from build123d import *

# Parameters (mm, degrees)
F0_R     = 2.5
F0_W     = 45
F0_H     = 50
F1_DEPTH = 3


# Not quite as in the source:
# - ends of sketch curves that miss each other by under 0.0002 mm in the source are joined


with BuildPart() as f1:
    # F0 (on Front) → F1 (new body)
    with BuildSketch(Plane.XZ):
        Polygon((72.0000029802, 36.0006778365), (72.0000029802, 50), (-72.0000029802, 50), (-72.0000029802, 36.0006778365), (-75.0000029802, 36.0006778365), (-75.0000029802, 21.7149635505), (-72.0000029802, 21.7149635505), (-72.0000029802, 7.4292492645), (-75.0000029802, 7.4292492645), (-75.0000029802, -6.8564650215), (-72.0000029802, -6.8564650215), (-72.0000029802, -21.1421793075), (-75.0000029802, -21.1421793075), (-75.0000029802, -35.4278935935), (-72.0000029802, -35.4278935935), (-72.0000029802, -46.7136078775), (-61.363272724, -46.7136078775), (-61.363272724, -49.7136078775), (-47.726909088, -49.7136078775), (-47.726909088, -46.7136078775), (-34.090545452, -46.7136078775), (-34.090545452, -49.7136078775), (-20.454181816, -49.7136078775), (-20.454181816, -46.7136078775), (-6.81781818, -46.7136078775), (-6.81781818, -49.7136078775), (6.818545456, -49.7136078775), (6.818545456, -46.7136078775), (20.454909092, -46.7136078775), (20.454909092, -49.7136078775), (34.091272728, -49.7136078775), (34.091272728, -46.7136078775), (47.727636364, -46.7136078775), (47.727636364, -49.7136078775), (61.364, -49.7136078775), (61.364, -46.7136078775), (72.0000029802, -46.7136078775), (72.0000029802, -35.4278935935), (75.0000029802, -35.4278935935), (75.0000029802, -21.1421793075), (72.0000029802, -21.1421793075), (72.0000029802, -6.8564650215), (75.0000029802, -6.8564650215), (75.0000029802, 7.4292492645), (72.0000029802, 7.4292492645), (72.0000029802, 21.7149635505), (75.0000029802, 21.7149635505), (75.0000029802, 36.0006778365), align=None)
        with Locations((-55.5279403925, -22.991552949)):
            Circle(F0_R, mode=Mode.SUBTRACT)
        with Locations((39.5000029802, -16.7136078775)):
            Rectangle(F0_W, F0_H, mode=Mode.SUBTRACT)
    extrude(amount=F1_DEPTH)


solid = f1.part
CAD build for the part. Positions are in the model's coordinates, mm. A direction names the side the tool comes from. Round coordinates to 2 decimals unless told otherwise and drop trailing zeros. Write each loop counter-clockwise with the first axis right and the second up, starting at its lowest first coordinate (ties: lowest second). Pieces come first, ordered by that corner, then holes. Notation, with made-up numbers: M 35.5,19.5 L 47.5,19.5 A22 ccw 47.5,31.5 Z; hole C -9,-19.75 d1. An arc over 180 degrees is marked long. Use a Markdown table: item, result. Add a question column.
1. Slice it at A-A on z = -5. Give the cut face in (x, y), then the cut area to 3 significant figures.
2. 3-axis set-ups, long thin cutter, end or side, ignore diameter. For faces 1 (the face through (-73, -1, 36.001)), 2 (the face through (74, -1, 7.429)), 3 (the face through (39, -1, -41.714)), 4 (the face through (-74, -1, -35.428)), 5 (the face through (-34.091, -1, -48)): which of +Z, -Z, +X, -X, +Y, -Y reach the whole face in a straight line?
3. Pull direction X, two halves, no side cores. Call faces 6 (the face through (72, -1, -14)), 7 (the face through (74, -1, 36.001)), 8 (the face through (-14, -1, -46.714)): released by +X, released by -X, zero draft, split by the parting line, or undercut.
4. Slice it at B-B on x = 55. Give the cut face in (y, z), then the cut area to 3 significant figures.
5. Slice it at C-C on x = 8.5. Give the cut face in (y, z).
6. Drill centre lines: probe 1 along X at (y, z) = (-0.9, -40); probe 2 along Z at (x, y) = (57, -1.1); probe 3 along Z at (x, y) = (45, -0.7). Where is each one in solid material? Low to high.
7. Slice it at D-D on y = -1.3. Give the number of separate pieces and of enclosed holes in the cut face, then the cut area to 3 significant figures.
8. Flat gauge pins, fed straight in: P1, Ø1.5, axis at x = -74, y = -1.5, coming from the -Z side; P2, Ø1.5, axis at y = -2, z = 17.5, coming from the -X side; P3, Ø0.9, axis at x = 73.5, y = -2, coming from the +Z side. Where does each tip first touch, or does it go through?
Reply:
| question | item | result |
|---|---|---|
| 1 | outline | M -75,-3 L 17,-3 L 17,0 L -75,0 Z; M 62,-3 L 75,-3 L 75,0 L 62,0 Z |
| 1 | area | 315 mm^2 |
| 2 | face 1 | +Z, -X, +Y, -Y |
| 2 | face 2 | +X, +Y, -Y |
| 2 | face 3 | +Y, -Y |
| 2 | face 4 | -Z, -X, +Y, -Y |
| 2 | face 5 | -Z, +Y, -Y |
| 3 | face 6 | released by +X |
| 3 | face 7 | zero draft |
| 3 | face 8 | undercut |
| 4 | outline | M -3,-49.71 L 0,-49.71 L 0,-41.71 L -3,-41.71 Z; M -3,8.29 L 0,8.29 L 0,50 L -3,50 Z |
| 4 | area | 149 mm^2 |
| 5 | outline | M -3,-46.71 L 0,-46.71 L 0,50 L -3,50 Z |
| 6 | probe 1 | x = -72 to 17, 62 to 72 |
| 6 | probe 2 | z = -49.71 to -41.71, 8.29 to 50 |
| 6 | probe 3 | z = -46.71 to -41.71, 8.29 to 50 |
| 7 | separate pieces | 1 |
| 7 | enclosed holes | 2 |
| 7 | area | 12,100 mm^2 |
| 8 | P1 | stops at z = -35.43 |
| 8 | P2 | stops at x = -72 |
| 8 | P3 | stops at z = 36 |
